The model under review builds one solid part; all positions refer to its coordinate system, in mm. A direction names the side the tool comes from. Coordinates: 2 decimals unless noted, no trailing zeros. Write each loop counter-clockwise with the first axis right and the second up, starting at its lowest first coordinate (ties: lowest second). Pieces come first, ordered by that corner, then holes. Notation, with made-up numbers: (34, -34) - (64, -34) arc R5 cw to (64, -27) - close; hole circle Ø10 at (-16.5, 79). An arc over 180 degrees is marked (long way). Put each result on its own line as item: value. Start each with the question number.
Item 1: Machinability: for faces 5 (the face through (-12, 15.1, -57.7)), 6 (the face through (-8, 0, -45)), which of the approach directions +Z, -Z, +X, -X, +Y, -Y give a long, thin tool a straight path to every point of the face, cutting with its end or side? Answer none if there is none.
Item 2: For pin 1 (1 mm diameter, centred on y = 9, z = -13, fed in from -X), flat-tipped, find the tip position at first contact; note if it passes through.
Item 3: Consider section D-D on y = 14. Give the boundary of the cut face in (x, z).
Item 4: Mouldability with a two-part tool opening along Y and no side actions: class faces 1 (the face through (-9.59, 24.1, -0.86)), 2 (the face through (-3.55, 16.86, -37.33)), 3 (the face through (-7.888, 17.664, -21.349)), 4 (the face through (-12, 20, -25.804)) as pulls with the +Y half, pulls with the -Y half, needs draft (parallel to the pull), parting line crosses it, or undercut.
Item 5: Consider section C-C on x = -13. Give the boundary of the cut face in (y, z).
Item 6: To check wall thickness, follow L1, parallel to Z at x = -3.25, y = 19.25; L2, parallel to Z at x = -5.25, y = 23.75; L3, parallel to X at y = 9.75, z = -6.5. State the ranges of each line that lie inside material, in increasing order. Write a range as [from, to].
Item 7: Consider section B-B on z = -6.5. Give the boundary of the cut face in (x, y), then the cut area to 3 significant figures.
Item 8: Consider section A-A on y = 2.5. Give the boundary of the cut face in (x, z), then the cut area to 3 significant figures.
Autodesk Inventor part; units mm, degrees
ref_plane "YZ Plane" through (0, 0, 0) normal (1, 0, 0) x (0, 1, 0)
ref_plane "XZ Plane" through (0, 0, 0) normal (0, 1, 0) x (-1, 0, 0)
ref_plane "XY Plane" through (0, 0, 0) normal (0, 0, 1) x (1, 0, 0)
sketch "Sketch1" plane through (0, 0, 0) normal (0, 1, 0) x (-1, 0, 0)
  line L0 (0, 0) -> (16, 0)
  line L1 (16, 0) -> (16, -91)
  line L2 (16, -91) -> (0, -91)
  line L3 (0, -91) -> (0, 0)
  dimension "d0" = 16
  dimension "d1" = 91
extrude "Extrusion1" add sketch "Sketch1" along normal blind 25
sketch "Sketch2" plane through (0, 25, 0) normal (0, 1, 0) x (1, 0, 0)
  line L0 (-16, 91) -> (-16, 0)
  circle A0 centre (-16, 12.8045) radius 4
  circle A1 centre (-16, 57.8045) radius 4
  point P0 (0, 0)
  dimension "d4" = 8
  dimension "d5" = 8
  dimension "d6" = 45
extrude "Extrusion2" cut sketch "Sketch2" against normal blind 20
fillet "Fillet1" radius 3 5 edges at (0, 12.5, -91) (0, 12.5, 0) (0, 25, -45.5) (-8, 25, -91) (-8, 25, 0)
sketch "Sketch3" plane through (0, 25, 0) normal (0, 1, 0) x (1, 0, 0)
  circle A0 centre (-7, 6.5) radius 2
  circle A1 centre (-7, 84.5) radius 2
  line L0 (-16, 8.8045) -> (-16, 3)
  line L1 (-16, 53.8045) -> (-16, 16.8045)
  line L2 (-16, 88) -> (-16, 61.8045)
  point P0 (0, 0)
  dimension "d10" = 4
  dimension "d12" = 4
  dimension "d15" = 9
  dimension "d17" = 9
  dimension "d18" = 6.5
sketch "Sketch4" plane through (0, 0, -3) normal (1, 0, 0) x (0, 0, -1)
  circle A0 centre (17.4261, 19.4387) radius 2
  circle A1 centre (69.9995, 19.4387) radius 2
  point P0 (-3, 0)
  dimension "d21" = 4
  dimension "d22" = 4
extrude "Extrusion4" cut sketch "Sketch4" against normal blind 30
sketch "Sketch5" plane through (-16, 0, -91) normal (-1, 0, 0) x (0, 0, 1)
  point P0 (91, 0)
sketch "Sketch6" plane through (-16, 0, -91) normal (-1, 0, 0) x (0, 0, 1)
  arc A0 (46.1955, 15) -> (65.1955, 15) centre (55.6955, 15) ccw
  line L0 (37.1955, 25) -> (37.1955, 5)
  line L1 (37.1955, 25) -> (74.1955, 25)
  line L2 (46.1955, 15) -> (46.1955, 30.0529)
  line L3 (46.1955, 30.0529) -> (65.1955, 30.0529)
  line L4 (65.1955, 30.0529) -> (65.1955, 15)
  point P0 (91, 0)
  dimension "d25" = 19
  dimension "d26" = 18.5
  dimension "d27" = 10
extrude "Extrusion5" cut sketch "Sketch6" against normal blind 9
sketch "Sketch7" plane through (-7, 0, -91) normal (-1, 0, 0) x (0, 0, 1)
  circle A0 centre (55.6955, 15) radius 2.75
  line L0 (37.1955, 25) -> (37.1955, 5)
  point P0 (91, 0)
  dimension "d30" = 5.5
  dimension "d31" = 18.5
extrude "Extrusion6" cut sketch "Sketch7" against normal blind 30
extrude "Extrusion7" cut sketch "Sketch3" against normal blind 30
properties part number "motorothersideradrod"
Report:
1. face 5: -X, +Y
1. face 6: +Z, -Z, +X, -X, -Y
2. pin 1: x = -12.06
3. outline: (-16, -91) - (-3, -91) arc R3 ccw to (0, -88) - (0, -37.87) - (-7, -37.87) - (-7, -44.75) - (-16, -44.75) - (-16, -53.8) arc R4 cw to (-16, -61.8) - close; (-16, -25.86) - (-7, -25.86) - (-7, -32.74) - (0, -32.74) - (0, -3) arc R3 ccw to (-3, 0) - (-16, 0) - (-16, -8.8) arc R4 cw to (-16, -16.8) - close; hole circle Ø4 at (-7, -84.5); hole circle Ø4 at (-7, -6.5)
4. face 1: pulls with the +Y half
4. face 2: undercut
4. face 3: undercut
4. face 4: needs draft
5. outline: (0, -91) - (22, -91) arc R3 ccw to (25, -88) - (25, -60.45) - (5, -60.45) - (5, -55.16) - (25, -55.16) - (25, -44.8) - (15, -44.8) arc R9.5 cw to (15, -25.8) - (25, -25.8) - (25, -15.45) - (5, -15.45) - (5, -10.16) - (25, -10.16) - (25, -3) arc R3 ccw to (22, 0) - (0, 0) - close; hole circle Ø4 at (19.44, -73); hole circle Ø4 at (19.44, -20.43)
6. L1: [-91, -74.99], [-71.01, -22.42], [-18.44, 0]
6. L2: [-90.44, -85.47], [-83.53, -7.47], [-5.53, -0.56]
6. L3: [-16, -9], [-5, 0]
7. outline: (-16, 0) - (-9, 0) - (-9, 25) - (-16, 25) - close; (-5, 0) - (0, 0) - (0, 22) arc R3 ccw to (-3, 25) - (-5, 25) - close
7. area: 298 mm²
8. outline: (-16, -91) - (-3, -91) arc R3 ccw to (0, -88) - (0, -3) arc R3 ccw to (-3, 0) - (-16, 0) - close; hole circle Ø4 at (-7, -84.5); hole circle Ø4 at (-7, -6.5)
8. area: 1,430 mm²
